from build123d import *

# Parameters (mm, degrees)
SKETCH1_W            = 75
SKETCH1_H            = 20
BOSS_EXTRUDE1_DEPTH  = 2
SKETCH2_W            = 62
SKETCH2_H            = 10
BOSS_EXTRUDE2_DEPTH  = 4
SKETCH3_W            = 70
SKETCH3_H            = 18
BOSS_EXTRUDE3_DEPTH  = 5
SKETCH4_W            = 6.142437882
SKETCH4_H            = 5.25340082
BOSS_EXTRUDE4_DEPTH  = 6
SKETCH6_W            = 2.181176029
SKETCH6_H            = 1.77174688
CUT_EXTRUDE1_DEPTH   = 6
LPATTERN1_COUNT      = 3
LPATTERN1_PITCH      = 12
LPATTERN1_COUNT_DIR2 = 3
LPATTERN1_PITCH_DIR2 = 12
CHAMFER1_SIZE        = 0.8
CHAMFER2_SIZE        = 1.5
CHAMFER4_SIZE        = 2


with BuildPart() as part:
    # Sketch1 → Boss-Extrude1 (new body)
    with BuildSketch(Plane.XY):
        Rectangle(SKETCH1_W, SKETCH1_H)
    extrude(amount=BOSS_EXTRUDE1_DEPTH)

    # Sketch2 → Boss-Extrude2 (add)
    with BuildSketch(Plane.XY.offset(2)):
        Rectangle(SKETCH2_W, SKETCH2_H)
    extrude(amount=BOSS_EXTRUDE2_DEPTH)

    # Sketch3 → Boss-Extrude3 (add)
    with BuildSketch(Plane(origin=(0, 0, 0), x_dir=(-1, 0, 0), z_dir=(0, 0, -1))):
        Rectangle(SKETCH3_W, SKETCH3_H)
    extrude(amount=BOSS_EXTRUDE3_DEPTH)

    # Sketch4 → Boss-Extrude4 (add)
    with BuildSketch(Plane.XY.offset(6)):
        Rectangle(SKETCH4_W, SKETCH4_H)
    boss_extrude4 = extrude(amount=BOSS_EXTRUDE4_DEPTH)

    # Sketch6 → Cut-Extrude1 (cut)
    with BuildSketch(Plane.XY.offset(12)):
        with Locations((1.290588015, 1.08587344)):
            Rectangle(SKETCH6_W, SKETCH6_H)
        with Locations((-1.290588015, 1.08587344)):
            Rectangle(SKETCH6_W, SKETCH6_H)
        with Locations((-1.290588015, -1.08587344)):
            Rectangle(SKETCH6_W, SKETCH6_H)
        with Locations((1.290588015, -1.08587344)):
            Rectangle(SKETCH6_W, SKETCH6_H)
    cut_extrude1 = extrude(amount=-CUT_EXTRUDE1_DEPTH, mode=Mode.SUBTRACT)

    # LPattern1: Boss-Extrude4, Cut-Extrude1 3 × 3
    with Locations(*[Vector(1, 0, 0) * (i * LPATTERN1_PITCH) + Vector(-1, 0, 0) * (j * LPATTERN1_PITCH_DIR2) for i in range(LPATTERN1_COUNT) for j in range(LPATTERN1_COUNT_DIR2) if (i, j) != (0, 0)]):
        add(boss_extrude4)
        add(cut_extrude1, mode=Mode.SUBTRACT)

    # Chamfer1
    chamfer1_edges = [part.edges().sort_by_distance(p)[0] for p in [
        (-15.071218941, -2.62670041, 9),
        (-27.071218941, -2.62670041, 9),
        (8.928781059, -2.62670041, 9),
        (20.928781059, -2.62670041, 9),
        (-3.071218941, -2.62670041, 9),
    ]]
    chamfer(chamfer1_edges, length=CHAMFER1_SIZE)

    # Chamfer2
    chamfer2_edges = [part.edges().sort_by_distance(p)[0] for p in [
        (31, -5, 4),
        (31, 5, 4),
        (-31, 5, 4),
        (-31, -5, 4),
    ]]
    chamfer(chamfer2_edges, length=CHAMFER2_SIZE)

    # Chamfer4
    chamfer4_edges = [part.edges().sort_by_distance(p)[0] for p in [
        (0, 10, 2),
        (37.5, 0, 2),
        (0, -10, 2),
        (-37.5, 0, 2),
    ]]
    chamfer(chamfer4_edges, length=CHAMFER4_SIZE - 0.0001)  # a hair under: the kernel refuses the full size


solid = part.part
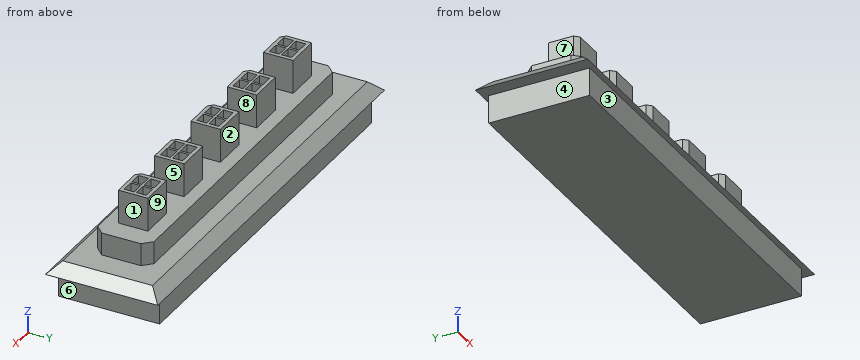
Part model, mm, in its own coordinate system. Face numbers are marked on the shaded views. A direction names the side the tool comes from. Coordinates: 2 decimals unless noted, no trailing zeros. Loops run counter-clockwise (first coordinate to the right, second up) from the corner with the lowest first, then second, coordinate; pieces in that order, holes last. Notation, with made-up numbers: (6, -21) -> (53, -21) arc R24 cw to (53, -5) -> close; hole circle Ø2 at (12, 63.25). An arc over 180 degrees is marked (long way). Use a Markdown table: item, result. Add a question column.
Item 1: Flat gauge pins, fed straight in: P1, Ø5, axis at y = 6.5, z = 7, coming from the +X side; P2, Ø2.5, axis at x = 13, z = 8, coming from the -Y side; P3, Ø1.4, axis at y = 1, z = 10.5, coming from the -X side. Where does each tip first touch, or does it go through?
Item 2: Band-saw the part on C-C on z = 5. Write the cut outline in (x, y).
Item 3: Which spindle directions (+Z, -Z, +X, -X, +Y, -Y) get a long thin tool onto all of the face, cutting with end or side? Do the marked faces 1, 2, 3, 4 and 5. Say none if no direction does.
Item 4: Probe probe 1 along Y at (x, z) = (-14, 10.75); probe 2 along Y at (x, z) = (-32.5, -4); probe 3 along Z at (x, y) = (24, -5.5). List the from-to ranges inside material, lowest first.
Item 5: Pull direction X, two halves, no side cores. Call the marked faces 6, 7, 8 and 9: +X half, -X half, draft (parallel to the pull), parting line (faces both ways), or undercut.
Geometry says:
| question | item | result |
|---|---|---|
| 1 | P1 | x = 30.29 |
| 1 | P2 | y = -2.63 |
| 1 | P3 | x = -27.07 |
| 2 | outline | (-31, -3.5) -> (-29.5, -5) -> (29.5, -5) -> (31, -3.5) -> (31, 3.5) -> (29.5, 5) -> (-29.5, 5) -> (-31, 3.5) -> close |
| 3 | face 1 | +Z, +X, +Y, -Y |
| 3 | face 2 | +Z, +X, -X, +Y |
| 3 | face 3 | -Z, +X, -X, -Y |
| 3 | face 4 | -Z, -X, +Y, -Y |
| 3 | face 5 | +Z, +Y, -Y |
| 4 | probe 1 | -2.63 to -1.97, -0.2 to 0.2, 1.97 to 2.63 |
| 4 | probe 2 | -9 to 9 |
| 4 | probe 3 | -5 to 2 |
| 5 | face 6 | +X half |
| 5 | face 7 | -X half |
| 5 | face 8 | undercut |
| 5 | face 9 | draft |
